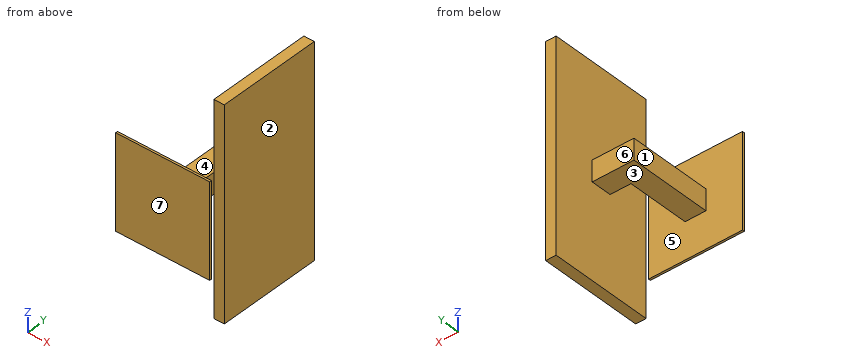
```python
from build123d import *

# Parameters (mm, degrees)
SKETCH2_W           = 45
SKETCH2_H           = 45
BOSS_EXTRUDE1_DEPTH = 1
SKETCH4_W           = 10
SKETCH4_H           = 10
BOSS_EXTRUDE3_DEPTH = 40
CUT_EXTRUDE4_DEPTH  = 30
BOSS_EXTRUDE8_DEPTH = 10
SKETCH18_W          = 100
SKETCH18_H          = 50
BOSS_EXTRUDE9_DEPTH = 5


with BuildPart() as part:
    # Sketch2 → Boss-Extrude1 (new body)
    with BuildSketch(Plane(origin=(0, 0, 0), x_dir=(1, 0, 0), z_dir=(0, 1, 0))):
        with Locations((22.5, 22.5)):
            Rectangle(SKETCH2_W, SKETCH2_H)
    extrude(amount=BOSS_EXTRUDE1_DEPTH)

    # Sketch4 → Boss-Extrude3 (add)
    with BuildSketch(Plane(origin=(0, 1, 0), x_dir=(1, 0, 0), z_dir=(0, 1, 0))):
        with Locations((22.5, 22.5)):
            Rectangle(SKETCH4_W, SKETCH4_H)
    extrude(amount=BOSS_EXTRUDE3_DEPTH)

    # Sketch10 → Cut-Extrude4 (cut)
    with BuildSketch(Plane(origin=(17.5, 41, -17.5), x_dir=(1, 0, 0), z_dir=(0, 0, 1))):
        Polygon((0, 0), (10, -9.949648776), (17.910752022, -1.998863577), (8.35816631, 7.505623697), align=None)
    extrude(amount=-CUT_EXTRUDE4_DEPTH, mode=Mode.SUBTRACT)

    # Sketch16 → Boss-Extrude8 (add)
    with BuildSketch(Plane(origin=(17.5, 41, -17.5), x_dir=(1, 0, 0), z_dir=(0, 0, 1))):
        Polygon((10, -9.949648776), (0, 0), (20, 0), (20, -9.949648776), align=None)
    extrude(amount=-BOSS_EXTRUDE8_DEPTH)

    # Sketch18 → Boss-Extrude9 (add)
    with BuildSketch(Plane(origin=(37.5, 0, 0), x_dir=(0, 0, -1), z_dir=(1, 0, 0))):
        with Locations((22.5, 36.025175612)):
            Rectangle(SKETCH18_W, SKETCH18_H)
    extrude(amount=BOSS_EXTRUDE9_DEPTH)


solid = part.part
```
Check sheet for the modelled part. Datum: model origin and axes. Units: mm. Face numbers are marked on the shaded views. A direction names the side the tool comes from. Round coordinates to 2 decimals unless told otherwise and drop trailing zeros. Loops run counter-clockwise (first coordinate to the right, second up) from the corner with the lowest first, then second, coordinate; pieces in that order, holes last. Notation, with made-up numbers: M -19.5,83 L 7.5,83 A24 cw 7.5,105 Z; hole C 81.5,77.5 d2. An arc over 180 degrees is marked long. Answer as a JSON object with one key per item and string values.
1. Mould release check, pull along Y, two halves, no side actions. Record for the marked faces 4, 5, 6 and 7: pulls with the +Y half, pulls with the -Y half, needs draft (parallel to the pull), parting line crosses it, or undercut.
Reply:
{"face 4": "needs draft", "face 5": "undercut", "face 6": "pulls with the +Y half", "face 7": "pulls with the -Y half"}
2. Section check A-A (y = 19). Record the boundary of the cut face in (x, z).
Reply:
{"outline": "M 17.5,-27.5 L 27.5,-27.5 L 27.5,-17.5 L 17.5,-17.5 Z; M 37.5,-72.5 L 42.5,-72.5 L 42.5,27.5 L 37.5,27.5 Z"}
3. Gauge pin test, flat ends, axial feed: P1, Ø5, axis at x = 16.5, y = 45, coming from the -Z side; P2, Ø2, axis at y = 20, z = -25.5, coming from the -X side; P3, Ø1.5, axis at x = 41, z = -38.5, coming from the -Y side; P4, Ø15, axis at y = 27.5, z = -39, coming from the +X side. Record the tip position at first contact, or that the pin passes through.
Reply:
{"P1": "passes through", "P2": "stops at x = 17.5", "P3": "stops at y = 0", "P4": "stops at x = 42.5"}
4. Section check B-B (z = -31.5). Record the boundary of the cut face in (x, y).
Reply:
{"outline": "M 0,0 L 45,0 L 45,1 L 0,1 Z; M 37.5,11.03 L 42.5,11.03 L 42.5,61.03 L 37.5,61.03 Z"}
5. Section check C-C (x = 26). Record the boundary of the cut face in (y, z).
Reply:
{"outline": "M 0,-45 L 1,-45 L 1,-27.5 L 41,-27.5 L 41,-17.5 L 1,-17.5 L 1,0 L 0,0 Z"}
6. Scan lines: line 1 (Y direction, x = 4, z = -0.5); line 2 (Z direction, x = 23, y = 14); line 3 (X direction, y = 23.5, z = -50.5). Record each from-to range of solid material in increasing order.
Reply:
{"line 1": "y = 0 to 1", "line 2": "z = -27.5 to -17.5", "line 3": "x = 37.5 to 42.5"}
7. Section check D-D (y = 39.5). Record the boundary of the cut face in (x, z), plus the area to 3 significant figures.
Reply:
{"outline": "M 17.5,-27.5 L 37.5,-27.5 L 37.5,-72.5 L 42.5,-72.5 L 42.5,27.5 L 37.5,27.5 L 37.5,-17.5 L 17.5,-17.5 Z", "area": "700 mm²"}
8. Access from +Z, -Z, +X, -X, +Y, -Y to the whole of each face (thin tool, end or side, straight path). Record for the marked faces 1, 2 and 3.
Reply:
{"face 1": "+Z, -Z, -X, +Y", "face 2": "+Z, -Z, +X, +Y", "face 3": "-Z, -X, +Y"}
